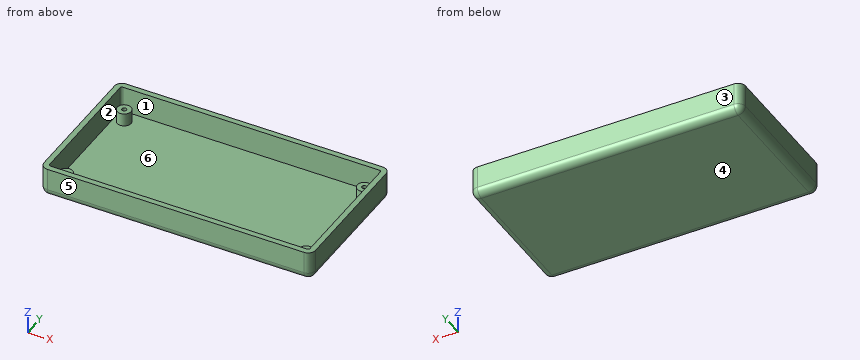
from build123d import *

# Parameters (mm, degrees)
SKETCH1_W           = 147
SKETCH1_H           = 78
BOSS_EXTRUDE1_DEPTH = 16
FILLET1_R           = 4
FILLET2_R           = 4
CUT_EXTRUDE1_DEPTH  = 14
SKETCH3_R           = 3.75
SKETCH3_R_2         = 1.25
BOSS_EXTRUDE2_DEPTH = 7


with BuildPart() as part:
    # Sketch1 → Boss-Extrude1 (new body)
    with BuildSketch(Plane.XY):
        Rectangle(SKETCH1_W, SKETCH1_H)
    extrude(amount=BOSS_EXTRUDE1_DEPTH)

    # Fillet1
    fillet1_edges = [part.edges().sort_by_distance(p)[0] for p in [
        (73.5, -39, 8),
        (-73.5, -39, 8),
        (-73.5, 39, 8),
        (73.5, 39, 8),
    ]]
    fillet(fillet1_edges, radius=FILLET1_R)

    # Fillet2
    fillet2_edges = [part.edges().sort_by_distance(p)[0] for p in [
        (0, -39, 0),
        (73.5, 0, 0),
        (-73.5, 0, 0),
        (0, 39, 0),
        (-72.328427125, 37.828427125, 0),
        (72.328427125, 37.828427125, 0),
        (72.328427125, -37.828427125, 0),
        (-72.328427125, -37.828427125, 0),
    ]]
    fillet(fillet2_edges, radius=FILLET2_R)

    # Sketch2 → Cut-Extrude1 (cut)
    with BuildSketch(Plane.XY.offset(16)):
        with BuildLine():
            Line((-70.5, 35), (-70.5, -35))
            ThreePointArc((-70.5, -35), (-70.207106781, -35.707106781), (-69.5, -36))
            Line((-69.5, -36), (69.5, -36))
            ThreePointArc((69.5, -36), (70.207106781, -35.707106781), (70.5, -35))
            Line((70.5, -35), (70.5, 35))
            ThreePointArc((70.5, 35), (70.207106781, 35.707106781), (69.5, 36))
            Line((69.5, 36), (-69.5, 36))
            ThreePointArc((-69.5, 36), (-70.207106781, 35.707106781), (-70.5, 35))
        make_face()
    extrude(amount=-CUT_EXTRUDE1_DEPTH, mode=Mode.SUBTRACT)

    # Sketch3 → Boss-Extrude2 (add)
    # profile 1 of 4: a face of its own
    with BuildSketch(Plane.XY.offset(2)):
        with Locations((-65, 29)):
            Circle(SKETCH3_R)
        with Locations((-65, 29)):
            Circle(SKETCH3_R_2, mode=Mode.SUBTRACT)
    # profile 2 of 4: a face of its own
    with BuildSketch(Plane.XY.offset(2)):
        with Locations(Location((65, 29, 0), (0, 0, 180))):
            Circle(SKETCH3_R)
        with Locations(Location((65, 29, 0), (0, 0, 180))):
            Circle(SKETCH3_R_2, mode=Mode.SUBTRACT)
    # profile 3 of 4: a face of its own
    with BuildSketch(Plane.XY.offset(2)):
        with Locations((65, -29)):
            Circle(SKETCH3_R)
        with Locations((65, -29)):
            Circle(SKETCH3_R_2, mode=Mode.SUBTRACT)
    # profile 4 of 4: a face of its own
    with BuildSketch(Plane.XY.offset(2)):
        with Locations(Location((-65, -29, 0), (0, 0, 180))):
            Circle(SKETCH3_R)
        with Locations(Location((-65, -29, 0), (0, 0, 180))):
            Circle(SKETCH3_R_2, mode=Mode.SUBTRACT)
    extrude(amount=BOSS_EXTRUDE2_DEPTH)


solid = part.part
Read the model definition and answer for the solid it produces. Units are mm, in the model's axes. Face numbers are marked on the shaded views. A direction names the side the tool comes from. Give positions to 0.01 mm unless a question says otherwise; leave off trailing zeros. Write each loop counter-clockwise with the first axis right and the second up, starting at its lowest first coordinate (ties: lowest second). Pieces come first, ordered by that corner, then holes. Notation, with made-up numbers: (78.5, 66.25) - (127.5, 66.25) arc R16 cw to (127.5, 93.25) - close; hole circle Ø1 at (54.5, 26.5). An arc over 180 degrees is marked (long way). Use CSV: the item, a comma, the result in double quotes. Start each with the question number.
Item 1: The part is cut by section C-C, the plane x = 2. Give the vertices of the cut face in (y, z), and give its area (3 significant figures).
Item 2: The part is cut by section B-B, the plane z = 14.25. Give the vertices of the cut face in (x, y).
Item 3: For the marked faces 5 and 6, determine the directions among +Z, -Z, +X, -X, +Y, -Y from which every point of the face is accessible in a straight line to the end or side of a thin tool.
Item 4: The part is cut by section A-A, the plane y = -21. Give the vertices of the cut face in (x, z), and give its area (3 significant figures).
Item 5: Consider line 1 (Y direction, x = 65, z = 5.75); line 2 (Y direction, x = -8.5, z = 5); line 3 (X direction, y = 32.5, z = 11). Determine where each line is inside the solid, lowest interval first.
Item 6: The mould has two halves that part along Y. Classify the marked faces 1, 2, 3 and 4: pulls with the +Y half, pulls with the -Y half, needs draft (parallel to the pull), parting line crosses it, or undercut.
Item 7: Flat-ended cylindrical pins translate along their axes: P1, Ø4, axis at x = 65, y = -29, coming from the +Z side; P2, Ø4, axis at x = -17.5, y = -1.5, coming from the +Z side. Find the tip coordinate at first contact, or state that the pin passes through.
Taken from the geometry:
1,outline,"(-39, 4) arc R4 ccw to (-35, 0) - (35, 0) arc R4 ccw to (39, 4) - (39, 16) - (36, 16) - (36, 2) - (-36, 2) - (-36, 16) - (-39, 16) - close"
1,area,"233 mm2"
2,outline,"(-73.5, -35) arc R4 ccw to (-69.5, -39) - (69.5, -39) arc R4 ccw to (73.5, -35) - (73.5, 35) arc R4 ccw to (69.5, 39) - (-69.5, 39) arc R4 ccw to (-73.5, 35) - close; hole (-70.5, -35) arc R1 ccw to (-69.5, -36) - (69.5, -36) arc R1 ccw to (70.5, -35) - (70.5, 35) arc R1 ccw to (69.5, 36) - (-69.5, 36) arc R1 ccw to (-70.5, 35) - close"
3,face 5,"+Z, -Z, +X, -X, -Y"
3,face 6,"+Z"
4,outline,"(-73.5, 4) arc R4 ccw to (-69.5, 0) - (69.5, 0) arc R4 ccw to (73.5, 4) - (73.5, 16) - (70.5, 16) - (70.5, 2) - (-70.5, 2) - (-70.5, 16) - (-73.5, 16) - close"
4,area,"371 mm2"
5,line 1,"-39 to -36, -32.75 to -30.25, -27.75 to -25.25, 25.25 to 27.75, 30.25 to 32.75, 36 to 39"
5,line 2,"-39 to -36, 36 to 39"
5,line 3,"-73.5 to -70.5, 70.5 to 73.5"
6,face 1,"undercut"
6,face 2,"undercut"
6,face 3,"pulls with the +Y half"
6,face 4,"needs draft"
7,P1,"z = 9"
7,P2,"z = 2"
